Check sheet for the modelled part. Datum: model origin and axes. Units: mm. A direction names the side the tool comes from. Coordinates: 2 decimals unless noted, no trailing zeros. Loops run counter-clockwise (first coordinate to the right, second up) from the corner with the lowest first, then second, coordinate; pieces in that order, holes last. Notation, with made-up numbers: M 39,-15 L 67,-15 A23 cw 67,-4 Z; hole C -20.5,-38.5 d3. An arc over 180 degrees is marked long. Answer in a Markdown table with one row per item. Add a question column.
```python
from build123d import *

# Parameters (mm, degrees)
F0_W     = 3.1658634543
F0_H     = 21.5854328126
F1_DEPTH = 15.494
F0_W_2   = 17.5561509095
F0_H_2   = 45.7611167803
F2_DEPTH = 25.4
F3_DEPTH = 25.4


with BuildPart() as f1:
    # F0 (on Front) → F1 (new body)
    with BuildSketch(Plane.XZ):
        Polygon((0, 10.7927164063), (-24.8951986432, 10.7927164063), (-24.8951986432, -10.7927164063), (4.1731842794, -10.7927164063), (4.1731842794, 10.7927164063), align=None)
        with Locations((23.312266916, 0)):
            Rectangle(F0_W, F0_H)
        Polygon((0, 62.3099505901), (0, 10.7927164063), (4.1731842794, 10.7927164063), (4.1731842794, 56.5538331866), (21.7293351889, 56.5538331866), (21.7293351889, 10.7927164063), (24.8951986432, 10.7927164063), (24.8951986432, 62.3099505901), align=None)
    extrude(amount=F1_DEPTH)

    # F0 (on Front) → F2 (join)
    with BuildSketch(Plane.XZ):
        with Locations((12.9512597341, 33.6732747965)):
            Rectangle(F0_W_2, F0_H_2)
    extrude(amount=F2_DEPTH)

    # F0 (on Front) → F3 (join)
    with BuildSketch(Plane.XZ):
        with Locations((12.9512597341, 0)):
            Rectangle(F0_W_2, F0_H)
    extrude(amount=F3_DEPTH)

    # F4: F1 across plane


with BuildPart() as f1_1:
    add(f1.part)
    add(f1.part.mirror(Plane.XZ))


solid = f1_1.part
```
Q1. Thickness scan on L1, parallel to Y at x = 23.5, z = 33; L2, parallel to Z at x = -9.5, y = -2.5; L3, parallel to X at y = -21, z = 7. Record the ranges inside material, lowest first.
Q2. Cross-section at C-C (y = -2). Record the cut outline in (x, z), plus the area to 3 significant figures.
Q3. Cross-section at A-A (z = 9). Record the cut outline in (x, y).
Q4. Cross-section at B-B (x = 15). Record the cut outline in (y, z).
Q5. Access from +Z, -Z, +X, -X, +Y, -Y to the whole of each face (thin tool, end or side, straight path). Record for faces 1 (the face through (-12, 0, 10.793)), 2 (the face through (21.729, -20, 22)), 3 (the face through (4.173, -20, 22)), 4 (the face through (13, -20, 56.554)), 5 (the face through (4.173, 20, 22)).
Q6. Go/stop test with flat-tipped pins: pin 1 (25 mm diameter, centred on x = -4, z = 41.5, fed in from +Y); pin 2 (8 mm diameter, centred on y = -0.5, z = 52, fed in from -X); pin 3 (5 mm diameter, centred on y = 19, z = 20, fed in from -X); pin 4 (3 mm diameter, centred on y = -23, z = 18.5, fed in from +X). Record where each tip stops, or that it passes through.
Q7. Cross-section at D-D (z = 17). Record the cut outline in (x, y), plus the area to 3 significant figures.
Answer key:
| question | item | result |
|---|---|---|
| 1 | L1 | -15.49 to 15.49 |
| 1 | L2 | -10.79 to 10.79 |
| 1 | L3 | 4.17 to 21.73 |
| 2 | outline | M -24.9,-10.79 L 24.9,-10.79 L 24.9,62.31 L 0,62.31 L 0,10.79 L -24.9,10.79 Z |
| 2 | area | 2,360 mm^2 |
| 3 | outline | M -24.9,-15.49 L 4.17,-15.49 L 4.17,-25.4 L 21.73,-25.4 L 21.73,-15.49 L 24.9,-15.49 L 24.9,15.49 L 21.73,15.49 L 21.73,25.4 L 4.17,25.4 L 4.17,15.49 L -24.9,15.49 Z |
| 4 | outline | M -25.4,-10.79 L 25.4,-10.79 L 25.4,56.55 L 15.49,56.55 L 15.49,62.31 L -15.49,62.31 L -15.49,56.55 L -25.4,56.55 Z |
| 5 | face 1 | +Z, -X, +Y, -Y |
| 5 | face 2 | +Z, -Z, +X, -Y |
| 5 | face 3 | +Z, -Z, -X, -Y |
| 5 | face 4 | +Z, +X, -X, -Y |
| 5 | face 5 | +Z, -Z, -X, +Y |
| 6 | pin 1 | y = 25.4 |
| 6 | pin 2 | x = 0 |
| 6 | pin 3 | x = 4.17 |
| 6 | pin 4 | x = 21.73 |
| 7 | outline | M 0,-15.49 L 4.17,-15.49 L 4.17,-25.4 L 21.73,-25.4 L 21.73,-15.49 L 24.9,-15.49 L 24.9,15.49 L 21.73,15.49 L 21.73,25.4 L 4.17,25.4 L 4.17,15.49 L 0,15.49 Z |
| 7 | area | 1,120 mm^2 |
